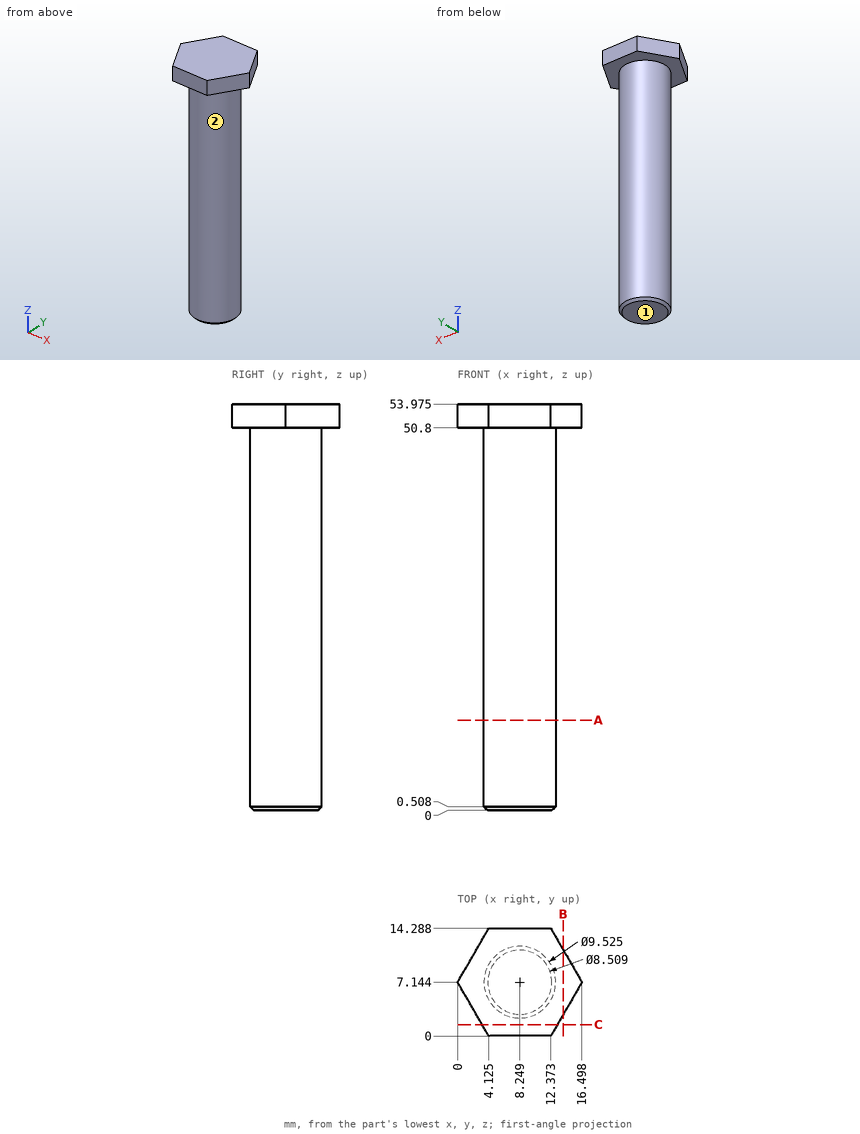
Can you work these out from the drawing? Everything is in mm from the part's minimum corner. A direction names the side the tool comes from. Coordinates: 2 decimals unless noted, no trailing zeros. Loops run counter-clockwise (first coordinate to the right, second up) from the corner with the lowest first, then second, coordinate; pieces in that order, holes last.
1. I need wall thicknesses on L1, parallel to Z at x = 15.25, y = 6 (1 decimal); L2, parallel to X at y = 7, z = 22; L3, parallel to Z at x = 3.75, y = 5.75 (1 decimal). Which ranges of each line are inside material? Lowest first, please.
2. Imagine slicing it at C-C, the plane y = 1.5. Please give me the cut outline in (x, z) (1 decimal).
3. Imagine slicing it at A-A, the plane z = 12. Please give me the cut outline in (x, y) (1 decimal).
4. Imagine slicing it at B-B, the plane x = 14. Please give me the cut outline in (y, z) (1 decimal).
5. For P1, Ø5, axis at y = 6.5, z = 9.5, coming from the +X side; P2, Ø1, axis at y = 6, z = 7.5, coming from the -X side; P3, Ø5, axis at y = 11, z = 40.5, coming from the -X side, each with a flat end and sliding along its axis, tell me the tip position at first contact or that it passes through.
6. For the marked faces 1 and 2, which set-ups out of +Z, -Z, +X, -X, +Y, -Y let a thin tool reach every point of the face, with its end or its side?
Taken from the geometry:
1. L1: z = 50.8 to 54
1. L2: x = 3.49 to 13.01
1. L3: z = 0.5 to 54
2. outline: (3.3, 50.8) - (13.2, 50.8) - (13.2, 54) - (3.3, 54) - close
3. outline: circle Ø9.5 at (8.2, 7.1)
4. outline: (2.8, 50.8) - (11.5, 50.8) - (11.5, 54) - (2.8, 54) - close
5. P1: stops at x = 13.01
5. P2: stops at x = 3.53
5. P3: stops at x = 3.68
6. face 1: -Z, +X, -X, +Y, -Y
6. face 2: -Z
